The listing builds one solid part. Answer for the finished solid, in the listing's coordinates (mm). A direction names the side the tool comes from. Give positions to 0.01 mm unless a question says otherwise; leave off trailing zeros. Loops run counter-clockwise (first coordinate to the right, second up) from the corner with the lowest first, then second, coordinate; pieces in that order, holes last. Notation, with made-up numbers: (15.5, 44) - (49.5, 44) arc R20 cw to (49.5, 55) - close; hole circle Ø4 at (19.5, 33.25). An arc over 180 degrees is marked (long way). Write item = value, one per line. Start each with the question number.
1) Consider probe 1 along X at (y, z) = (0, -10); probe 2 along Z at (x, y) = (-0.7, 0); probe 3 along X at (y, z) = (-0.75, -7). Determine where each line is inside the solid, lowest interval first.
2) The part is cut by section C-C on y = 7.5. Write down the section's boundary in (x, z).
3) The part is cut by section A-A on x = 11. Write down the section's boundary in (y, z).
4) Flat-ended cylindrical pins translate along their axes: P1, Ø6, axis at y = -7, z = -12, coming from the +X side; P2, Ø2.5, axis at y = 0, z = -20, coming from the -X side; P3, Ø4, axis at y = 1, z = -17, coming from the +X side. Find the tip coordinate at first contact, or state that the pin passes through.
5) The mould has two halves that part along Z. Classify faces 4 (the cylindrical face through (-0.81, 8.05, 23.57)), 5 (the cylindrical face through (-0.81, 8.05, -23.57)), 6 (the cylindrical face through (-0.789, -0.208, -18.414)), 7 (the flat face through (0, 4, 0)): +Z half, -Z half, draft (parallel to the pull), parting line (faces both ways), or undercut.
6) The part is cut by section B-B on y = 0. State how many separate pieces and enclosed holes the cut face has, plus the area to 3 significant figures.
7) Which of the six approach directions +Z, -Z, +X, -X, +Y, -Y give full straight-line access (tool end or side, diameter ignored) to faces 1 (the cylindrical face through (-0.789, -0.208, 21.586)), 2 (the cylindrical face through (5.776, 1.29, -2.024)), 3 (the flat face through (-1, 0, -25))?
from build123d import *

# Parameters (mm, degrees)
F1_R     = 2.4
F3_W     = 19.1
F3_H     = 50
F3_R     = 1.6
F4_DEPTH = 1.6
F5_R     = 5
F6_R     = 1


with BuildPart() as f2:
    # F2: sweep along a path in F0
    with BuildLine(Plane.XZ) as f2_path:
        ThreePointArc((43.4729635533, 19.6961550602), (55.2614034679, -12.9263128614), (21.1438191684, -6.6666666667))
        ThreePointArc((21.1438191684, -6.6666666667), (17.4892314444, -1.8350341907), (11.7157287525, 0))
        Line((11.7157287525, 0), (0, 0))
    # F1 (on Right) → F2 (sweep)
    with BuildSketch(Plane.YZ):
        Circle(F1_R)
    sweep(path=f2_path.line)

    # F3 (on Right) → F4 (join)
    with BuildSketch(Plane.YZ):
        Rectangle(F3_W, F3_H)
        with Locations((0, -20)):
            Circle(F3_R, mode=Mode.SUBTRACT)
        with Locations((0, 20)):
            Circle(F3_R, mode=Mode.SUBTRACT)
    extrude(amount=-F4_DEPTH)

    # F5
    f5_edges = [f2.edges().sort_by_distance(p)[0] for p in [
        (-0.8, -9.55, 25),
        (-0.8, 9.55, 25),
        (-0.8, -9.55, -25),
        (-0.8, 9.55, -25),
    ]]
    fillet(f5_edges, radius=F5_R)

    # F6
    f6_edges = [f2.edges().sort_by_distance(p)[0] for p in [
        (43.472964, -2.4, 19.696155),
    ]]
    fillet(f6_edges, radius=F6_R)


solid = f2.part
Answer below:
q1.probe_1 = -1.6 to 0, 19.96 to 25.52, 54.48 to 60.04
q1.probe_2 = -25 to -21.6, -18.4 to 18.4, 21.6 to 25
q1.probe_3 = -1.6 to 0, 18.83 to 23.72, 56.28 to 61.15
q2.outline = (-1.6, -24.04) - (0, -24.04) - (0, 24.04) - (-1.6, 24.04) - close
q3.outline = circle Ø4.8 at (0, 0)
q4.P1 = 0
q4.P2 = 27.74
q4.P3 = 56.51
q5.face_4 = +Z half
q5.face_5 = -Z half
q5.face_6 = undercut
q5.face_7 = draft
q6.separate_pieces = 3
q6.enclosed_holes = 0
q6.area = 588 mm2
q7.face_1 = -X
q7.face_2 = none
q7.face_3 = -Z, +X, -X, +Y, -Y
